Drawing for the job (mm, zero at the part's lowest x, y, z). A direction names the side the tool comes from. Round coordinates to 2 decimals unless told otherwise and drop trailing zeros. Write each loop counter-clockwise with the first axis right and the second up, starting at its lowest first coordinate (ties: lowest second). Pieces come first, ordered by that corner, then holes.
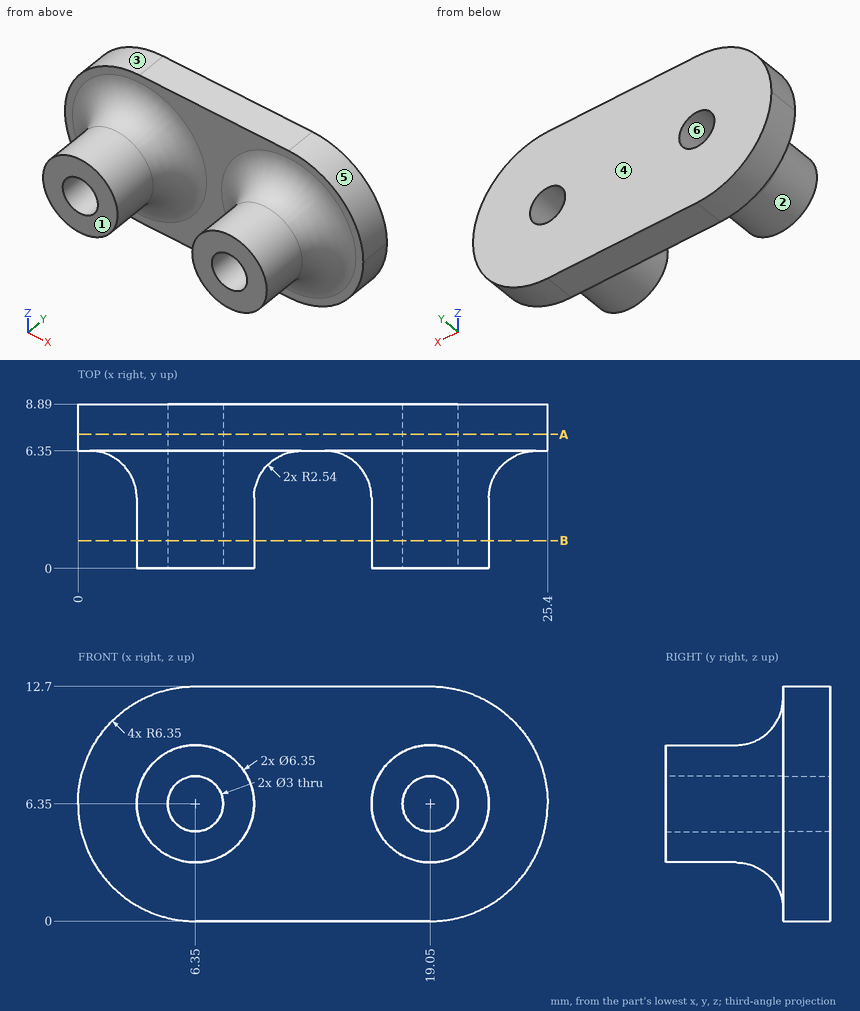
Q1. Saw through at A-A, the plane y = 7.25. Give the number of separate pieces and of enclosed holes in the cut face, and give its area (3 significant figures).
Q2. Tool access for the marked faces 1 and 2: list every direction of +Z, -Z, +X, -X, +Y, -Y with a clear straight run to the whole face (end or side of a thin tool).
Q3. Drop flat-ended pins along their axis: P1, Ø2, axis at x = 12, z = 7.5, coming from the -Y side; P2, Ø1.5, axis at y = 5, z = 3.5, coming from the +X side; P3, Ø2, axis at y = 2.5, z = 7, coming from the +X side (3 decimals). Give the stop position or say it passes through.
Q4. Saw through at B-B, the plane y = 1.5. Write the cut outline in (x, z) (3 decimals), and give its area (3 significant figures).
Q5. Wall check: line 1 (X direction, y = 6.5, z = 6.35); line 2 (Z direction, x = 19.05, y = 7); line 3 (X direction, y = 2, z = 5.5). Give the ranges that are in metal, low to high.
Q6. Two-plate mould, pull along X, no slides. Class the marked faces 3, 4, 5 and 6: released by +X, released by -X, zero draft, split by the parting line, or undercut.
Computed:
1. separate pieces: 1
1. enclosed holes: 2
1. area: 274 mm2
2. face 1: +Z, -Z, +X, -X, -Y
2. face 2: -Y
3. P1: stops at y = 6.17
3. P2: stops at x = 22.15
3. P3: stops at x = 22.225
4. outline: circle Ø6.35 at (6.35, 6.35); circle Ø6.35 at (19.05, 6.35); hole circle Ø3 at (6.35, 6.35); hole circle Ø3 at (19.05, 6.35)
4. area: 49.2 mm2
5. line 1: x = 0 to 4.85, 7.85 to 17.55, 20.55 to 25.4
5. line 2: z = 0 to 4.85, 7.85 to 12.7
5. line 3: x = 3.29 to 5.11, 7.59 to 9.41, 15.99 to 17.81, 20.29 to 22.11
6. face 3: released by -X
6. face 4: zero draft
6. face 5: released by +X
6. face 6: undercut
